from build123d import *

# Parameters (mm, degrees)
SKETCH_1_R       = 1.65
F_3MM_DEPTH      = 3
F_32MM_1_START   = 3
F_32MM_1_DEPTH   = 8
F_32MM_1_2_DEPTH = 8


with BuildPart() as part:
    # 草图1 → 斜切鼻件底座_3mm (new body)
    with BuildSketch(Plane.XY):
        Polygon((-29, 73), (29, 73), (44, 76), (36, 82), (20, 91), (-20, 91), (-36, 82), (-44, 76), align=None)
        with Locations((-12, 89)):
            Circle(SKETCH_1_R, mode=Mode.SUBTRACT)
        with Locations((12, 89)):
            Circle(SKETCH_1_R, mode=Mode.SUBTRACT)
    extrude(amount=F_3MM_DEPTH)

    # 草图2 → 32mm__-1 (add)
    with BuildSketch(Plane.XY.offset(F_32MM_1_START)):
        Polygon((-27, 73), (-17, 73), (-16, 74), (-16, 76), (-17, 77), (-27, 77), (-28, 76), (-28, 74), align=None)
    extrude(amount=F_32MM_1_DEPTH)

    # 草图3 → 32mm__1 2 (add)
    with BuildSketch(Plane.XY.offset(F_32MM_1_START)):
        Polygon((17, 73), (27, 73), (28, 74), (28, 76), (27, 77), (17, 77), (16, 76), (16, 74), align=None)
    extrude(amount=F_32MM_1_2_DEPTH)


solid = part.part
Could you check a few things on this model? Use its own coordinates, in mm. A direction names the side the tool comes from. Round coordinates to 2 decimals unless told otherwise and drop trailing zeros. Loops run counter-clockwise (first coordinate to the right, second up) from the corner with the lowest first, then second, coordinate; pieces in that order, holes last. Notation, with made-up numbers: (-37.5, 27.5) -> (-33.5, 27.5) arc R16 ccw to (-33.5, 53.5) -> close; hole circle Ø11 at (84.5, 2). An arc over 180 degrees is marked (long way). Use CSV: the item, a comma, the result in double quotes.
(1) If we mould it in two halves opening along X, with no side actions, what happens to faces 1 (the flat face through (28.11, 86.44, 1.48)), 2 (the flat face through (0, 73, 2)), 3 (the cylindrical face through (-12.4, 87.4, 1.5))? For each: +X half, -X half, draft (parallel to the pull), parting line (faces both ways), or undercut.
Return value:
face 1,"+X half"
face 2,"draft"
face 3,"undercut"
(2) Suppose I cut it at B-B on x = 12. Write out the boundary of the cut face in (y, z), plus the area to 3 significant figures.
Return value:
outline,"(73, 0) -> (87.35, 0) -> (87.35, 3) -> (73, 3) -> close; (90.65, 0) -> (91, 0) -> (91, 3) -> (90.65, 3) -> close"
area,"44.1 mm²"
(3) If I drill on probe 1 along X at (y, z) = (89, 0.75); probe 2 along Y at (x, z) = (12, 0.7); probe 3 along Z at (x, y) = (1.5, 76.5), over which ranges is the centre line in solid material (lowest first)? Write a range as [from, to].
Return value:
probe 1,"x = [-23.56, -13.65], [-10.35, 10.35], [13.65, 23.56]"
probe 2,"y = [73, 87.35], [90.65, 91]"
probe 3,"z = [0, 3]"
(4) Will these pins go through, and if not, where does the flat tip stop? pin 1 Ø2 at (y, z) = (75, 5) entering from +X; pin 2 Ø2.5 at (x, z) = (19.5, 7) entering from +Y; pin 3 Ø2.5 at (x, y) = (12, 89) entering from -Z; pin 4 Ø2 at (x, y) = (-6, 88.5) entering from +Z.
Return value:
pin 1,"stops at x = 28"
pin 2,"stops at y = 77"
pin 3,"passes through"
pin 4,"stops at z = 3"
(5) Suppose I cut it at A-A on z = 10.25. Write out the boundary of the cut face in (x, y), plus the area to 3 significant figures.
Return value:
outline,"(-28, 74) -> (-27, 73) -> (-17, 73) -> (-16, 74) -> (-16, 76) -> (-17, 77) -> (-27, 77) -> (-28, 76) -> close; (16, 74) -> (17, 73) -> (27, 73) -> (28, 74) -> (28, 76) -> (27, 77) -> (17, 77) -> (16, 76) -> close"
area,"92.0 mm²"
(6) Suppose I cut it at C-C on z = 1.25. Write out the boundary of the cut face in (x, y).
Return value:
outline,"(-44, 76) -> (-29, 73) -> (29, 73) -> (44, 76) -> (36, 82) -> (20, 91) -> (-20, 91) -> (-36, 82) -> close; hole circle Ø3.3 at (-12, 89); hole circle Ø3.3 at (12, 89)"
(7) Suppose I cut it at D-D on y = 89. Write out the boundary of the cut face in (x, z), plus the area to 3 significant figures.
Return value:
outline,"(-23.56, 0) -> (-13.65, 0) -> (-13.65, 3) -> (-23.56, 3) -> close; (-10.35, 0) -> (10.35, 0) -> (10.35, 3) -> (-10.35, 3) -> close; (13.65, 0) -> (23.56, 0) -> (23.56, 3) -> (13.65, 3) -> close"
area,"122 mm²"
(8) For faces 4 (the flat face through (-28, 75, 7)), 5 (the flat face through (22, 77, 7)), 6 (the flat face through (28, 75, 7)), which set-ups out of +Z, -Z, +X, -X, +Y, -Y let a thin tool reach every point of the face, with its end or its side?
Return value:
face 4,"+Z, -X, +Y, -Y"
face 5,"+Z, +X, -X, +Y"
face 6,"+Z, +X, +Y, -Y"
